```python
from build123d import *

# Parameters (mm, degrees)
F0_R     = 61.5
F1_DEPTH = 25


with BuildPart() as f1:
    # F0 (on Front) → F1 (new body)
    with BuildSketch(Plane.XZ):
        Circle(F0_R)
        with BuildLine():
            ThreePointArc((-28.054004, -53.546012), (-13.904054, -56.461066), (0, -52.537306))
            ThreePointArc((0, -52.537306), (13.904054, -56.461066), (28.054004, -53.546012))
            ThreePointArc((28.054004, -53.546012), (0, -60.45), (-28.054004, -53.546012))
        make_face(mode=Mode.SUBTRACT)
        with BuildLine():
            ThreePointArc((-44.487497, -26.839569), (-29.986229, -30.499997), (-15.488273, -26.826475))
            ThreePointArc((-15.488273, -26.826475), (-11.420658, -41.218834), (-1, -51.947086))
            ThreePointArc((-1, -51.947086), (-29.75, -51.528512), (-44.487497, -26.839569))
        make_face(mode=Mode.SUBTRACT)
        with BuildLine():
            ThreePointArc((0, -51.382534), (-10.404205, -40.976641), (-14.487497, -26.839569))
            ThreePointArc((-14.487497, -26.839569), (0, -30.5), (14.487497, -26.839569))
            ThreePointArc((14.487497, -26.839569), (10.404205, -40.976641), (0, -51.382534))
        make_face(mode=Mode.SUBTRACT)
        with BuildLine():
            ThreePointArc((-60.399208, -2.477526), (-55.848744, -16.189269), (-45.498641, -26.268653))
            ThreePointArc((-45.498641, -26.268653), (-41.94469, -40.271797), (-32.345204, -51.068486))
            ThreePointArc((-32.345204, -51.068486), (-52.351236, -30.225), (-60.399208, -2.477526))
        make_face(mode=Mode.SUBTRACT)
        with BuildLine():
            ThreePointArc((-45.487042, 25.091798), (-41.402951, 10.71203), (-30.976545, 0))
            ThreePointArc((-30.976545, 0), (-41.406887, -10.718838), (-45.487497, -25.107518))
            ThreePointArc((-45.487497, -25.107518), (-59.487041, -0.007733), (-45.487042, 25.091798))
        make_face(mode=Mode.SUBTRACT)
        with BuildLine():
            ThreePointArc((-44.498586, -25.691944), (-40.689081, -11.47831), (-30.487497, -0.873244))
            ThreePointArc((-30.487497, -0.873244), (-26.409976, -15.256598), (-15.987047, -25.974321))
            ThreePointArc((-15.987047, -25.974321), (-30.279198, -29.50655), (-44.498586, -25.691944))
        make_face(mode=Mode.SUBTRACT)
        with BuildLine():
            ThreePointArc((-29.487497, -0.858807), (-17.326184, -4.430401), (-4.76314, -2.75))
            ThreePointArc((-4.76314, -2.75), (-12.499932, -12.789714), (-15.487497, -25.107518))
            ThreePointArc((-15.487497, -25.107518), (-25.547749, -14.75), (-29.487497, -0.858807))
        make_face(mode=Mode.SUBTRACT)
        with BuildLine():
            ThreePointArc((-14.473642, -25.099514), (-10.534797, -11.238761), (-0.500455, -0.897245))
            ThreePointArc((-0.500455, -0.897245), (-4.439299, -14.757998), (-14.473642, -25.099514))
        make_face(mode=Mode.SUBTRACT)
        with BuildLine():
            ThreePointArc((1, -51.947086), (11.420658, -41.218834), (15.488273, -26.826475))
            ThreePointArc((15.488273, -26.826475), (29.986229, -30.499997), (44.487497, -26.839569))
            ThreePointArc((44.487497, -26.839569), (29.75, -51.528512), (1, -51.947086))
        make_face(mode=Mode.SUBTRACT)
        with BuildLine():
            ThreePointArc((-14, -25.966324), (-4.826252, -17.220116), (0, -5.5))
            ThreePointArc((0, -5.5), (4.826252, -17.220116), (14, -25.966324))
            ThreePointArc((14, -25.966324), (0, -29.5), (-14, -25.966324))
        make_face(mode=Mode.SUBTRACT)
        with BuildLine():
            ThreePointArc((14.486594, -25.091517), (4.452251, -14.75), (0.513406, -0.889245))
            ThreePointArc((0.513406, -0.889245), (10.547749, -11.230762), (14.486594, -25.091517))
        make_face(mode=Mode.SUBTRACT)
        with BuildLine():
            ThreePointArc((28.973189, 0), (15, -3.519238), (1.026811, 0))
            ThreePointArc((1.026811, 0), (15, 3.519238), (28.973189, 0))
        make_face(mode=Mode.SUBTRACT)
        with BuildLine():
            ThreePointArc((15.487497, -25.107518), (12.499932, -12.789714), (4.76314, -2.75))
            ThreePointArc((4.76314, -2.75), (17.326184, -4.430401), (29.487497, -0.858807))
            ThreePointArc((29.487497, -0.858807), (25.547749, -14.75), (15.487497, -25.107518))
        make_face(mode=Mode.SUBTRACT)
        with BuildLine():
            ThreePointArc((44.498579, -25.691267), (30.28471, -29.498626), (16, -25.966324))
            ThreePointArc((16, -25.966324), (26.413775, -15.25), (30.487497, -0.873244))
            ThreePointArc((30.487497, -0.873244), (40.688914, -11.478015), (44.498579, -25.691267))
        make_face(mode=Mode.SUBTRACT)
        with BuildLine():
            ThreePointArc((32.345204, -51.068486), (41.94469, -40.271797), (45.498641, -26.268653))
            ThreePointArc((45.498641, -26.268653), (55.848744, -16.189269), (60.399208, -2.477526))
            ThreePointArc((60.399208, -2.477526), (52.351236, -30.225), (32.345204, -51.068486))
        make_face(mode=Mode.SUBTRACT)
        with BuildLine():
            ThreePointArc((-32.345204, 51.068486), (-41.94469, 40.271797), (-45.498641, 26.268653))
            ThreePointArc((-45.498641, 26.268653), (-55.848744, 16.189269), (-60.399208, 2.477526))
            ThreePointArc((-60.399208, 2.477526), (-52.351236, 30.225), (-32.345204, 51.068486))
        make_face(mode=Mode.SUBTRACT)
        with BuildLine():
            ThreePointArc((-44.498426, 25.676034), (-30.286966, 29.490471), (-16.000887, 25.965778))
            ThreePointArc((-16.000887, 25.965778), (-26.414035, 15.249549), (-30.487497, 0.873244))
            ThreePointArc((-30.487497, 0.873244), (-40.685169, 11.471382), (-44.498426, 25.676034))
        make_face(mode=Mode.SUBTRACT)
        with BuildLine():
            ThreePointArc((-15.487497, 25.107518), (-12.499932, 12.789714), (-4.76314, 2.75))
            ThreePointArc((-4.76314, 2.75), (-17.326184, 4.430401), (-29.487497, 0.858807))
            ThreePointArc((-29.487497, 0.858807), (-25.547749, 14.75), (-15.487497, 25.107518))
        make_face(mode=Mode.SUBTRACT)
        with BuildLine():
            ThreePointArc((-28.973189, 0), (-15, 3.519238), (-1.026811, 0))
            ThreePointArc((-1.026811, 0), (-15, -3.519238), (-28.973189, 0))
        make_face(mode=Mode.SUBTRACT)
        with BuildLine():
            ThreePointArc((-14.486594, 25.091517), (-4.443107, 14.74859), (-0.500455, 0.881244))
            ThreePointArc((-0.500455, 0.881244), (-10.543942, 11.224172), (-14.486594, 25.091517))
        make_face(mode=Mode.SUBTRACT)
        with BuildLine():
            ThreePointArc((-1, 51.947086), (-11.420658, 41.218834), (-15.488273, 26.826475))
            ThreePointArc((-15.488273, 26.826475), (-29.986229, 30.499997), (-44.487497, 26.839569))
            ThreePointArc((-44.487497, 26.839569), (-29.75, 51.528512), (-1, 51.947086))
        make_face(mode=Mode.SUBTRACT)
        with BuildLine():
            ThreePointArc((-2e-06, 51.382535), (10.404204, 40.976642), (14.487497, 26.839569))
            ThreePointArc((14.487497, 26.839569), (0, 30.5), (-14.487497, 26.839569))
            ThreePointArc((-14.487497, 26.839569), (-10.404206, 40.976641), (-2e-06, 51.382535))
        make_face(mode=Mode.SUBTRACT)
        with BuildLine():
            ThreePointArc((14.486594, 25.091517), (10.547749, 11.230762), (0.513406, 0.889245))
            ThreePointArc((0.513406, 0.889245), (4.452251, 14.75), (14.486594, 25.091517))
        make_face(mode=Mode.SUBTRACT)
        with BuildLine():
            ThreePointArc((29.487497, 0.858807), (17.326184, 4.430401), (4.76314, 2.75))
            ThreePointArc((4.76314, 2.75), (12.499932, 12.789714), (15.487497, 25.107518))
            ThreePointArc((15.487497, 25.107518), (25.547749, 14.75), (29.487497, 0.858807))
        make_face(mode=Mode.SUBTRACT)
        with BuildLine():
            ThreePointArc((44.498579, 25.691267), (40.688914, 11.478016), (30.487496, 0.873246))
            ThreePointArc((30.487496, 0.873246), (26.413774, 15.250001), (16, 25.966324))
            ThreePointArc((16, 25.966324), (30.28471, 29.498626), (44.498579, 25.691267))
        make_face(mode=Mode.SUBTRACT)
        with BuildLine():
            ThreePointArc((-14, 25.966324), (0, 29.5), (14, 25.966324))
            ThreePointArc((14, 25.966324), (4.826252, 17.220116), (0, 5.5))
            ThreePointArc((0, 5.5), (-4.826252, 17.220116), (-14, 25.966324))
        make_face(mode=Mode.SUBTRACT)
        with BuildLine():
            ThreePointArc((45.487497, -25.107518), (41.406887, -10.718838), (30.976545, 0))
            ThreePointArc((30.976545, 0), (41.406887, 10.718838), (45.487497, 25.107518))
            ThreePointArc((45.487497, 25.107518), (59.5, 0), (45.487497, -25.107518))
        make_face(mode=Mode.SUBTRACT)
        with BuildLine():
            ThreePointArc((60.399208, 2.477526), (55.848744, 16.189269), (45.498641, 26.268653))
            ThreePointArc((45.498641, 26.268653), (41.94469, 40.271797), (32.345204, 51.068486))
            ThreePointArc((32.345204, 51.068486), (52.351236, 30.225), (60.399208, 2.477526))
        make_face(mode=Mode.SUBTRACT)
        with BuildLine():
            ThreePointArc((44.487497, 26.839569), (29.986229, 30.499997), (15.488273, 26.826475))
            ThreePointArc((15.488273, 26.826475), (11.420657, 41.218835), (0.999998, 51.947088))
            ThreePointArc((0.999998, 51.947088), (29.75, 51.528514), (44.487497, 26.839569))
        make_face(mode=Mode.SUBTRACT)
        with BuildLine():
            ThreePointArc((28.054004, 53.546012), (13.904054, 56.461066), (0, 52.537306))
            ThreePointArc((0, 52.537306), (-13.904054, 56.461066), (-28.054004, 53.546012))
            ThreePointArc((-28.054004, 53.546012), (0, 60.45), (28.054004, 53.546012))
        make_face(mode=Mode.SUBTRACT)
    extrude(amount=F1_DEPTH)


solid = f1.part
```
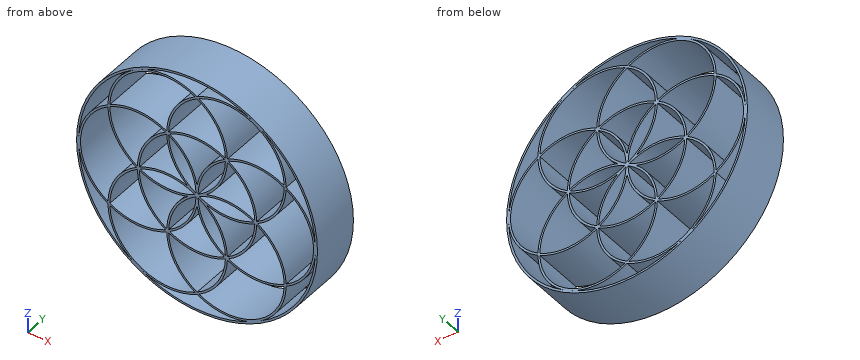
The listing builds one solid part. Answer for the finished solid, in the listing's coordinates (mm). Coordinates: 2 decimals unless noted, no trailing zeros. Loops run counter-clockwise (first coordinate to the right, second up) from the corner with the lowest first, then second, coordinate; pieces in that order, holes last. Notation, with made-up numbers: M 11.25,21.5 L 57.25,21.5 A13 ccw 57.25,46.5 Z; hole C 8,88 d7. An arc over 180 degrees is marked long. Answer as a JSON object with one key per item and string values. Group by question number.
Item 1: Section D-D (z = -41) is taken. Write down the section's boundary in (x, y).
Item 2: Section C-C (x = 53.5) is taken. Write down the section's boundary in (y, z), and give its area (3 significant figures).
Item 3: Section B-B (x = 37) is taken. Give the number of separate pieces and of enclosed holes in the cut face, and give its area (3 significant figures).
Item 4: Section A-A (z = 46) is taken. Write down the section's boundary in (x, y).
Item 5: Consider L1, parallel to X at y = -10.5, z = 47; L2, parallel to Z at x = -50, y = -10.5; L3, parallel to Z at x = -48, y = -23. Determine where each line is inside the solid, lowest interval first.
Item 6: Each of these flat-tipped pins is pushed along its axis until it touches: P1, Ø12, axis at y = -11.5, z = -14.5, coming from the -X side; P2, Ø10, axis at y = -18, z = -46, coming from the -X side; P3, Ø6, axis at y = -3.5, z = 33, coming from the -X side. Where does it stop, or does it pass through?
Solved:
{
 "1": {"outline": "M -45.84,-25 L -44.42,-25 L -44.42,0 L -45.84,0 Z; M -41.55,-25 L -40.39,-25 L -40.39,0 L -41.55,0 Z; M -11.55,-25 L -10.39,-25 L -10.39,0 L -11.55,0 Z; M 10.39,-25 L 11.55,-25 L 11.55,0 L 10.39,0 Z; M 40.39,-25 L 41.55,-25 L 41.55,0 L 40.39,0 Z; M 44.42,-25 L 45.84,-25 L 45.84,0 L 44.42,0 Z"},
 "2": {"outline": "M -25,-30.33 L 0,-30.33 L 0,-28.14 L -25,-28.14 Z; M -25,-19.44 L 0,-19.44 L 0,-17.83 L -25,-17.83 Z; M -25,17.83 L 0,17.83 L 0,19.44 L -25,19.44 Z; M -25,28.14 L 0,28.14 L 0,30.33 L -25,30.33 Z", "area": "190 mm2"},
 "3": {"separate pieces": "8", "enclosed holes": "0", "area": "265 mm2"},
 "4": {"outline": "M -40.82,-25 L -39.22,-25 L -39.22,0 L -40.82,0 Z; M -38.01,-25 L -36.67,-25 L -36.67,0 L -38.01,0 Z; M -8.01,-25 L -6.67,-25 L -6.67,0 L -8.01,0 Z; M 6.67,-25 L 8.01,-25 L 8.01,0 L 6.67,0 Z; M 36.67,-25 L 38.01,-25 L 38.01,0 L 36.67,0 Z; M 39.22,-25 L 40.82,-25 L 40.82,0 L 39.22,0 Z"},
 "5": {"L1": "x = -39.66 to -38.02, -37.1 to -35.7, -7.1 to -5.7, 5.7 to 7.1, 35.7 to 37.1, 38.02 to 39.66", "L2": "z = -35.81 to -33.97, -23.03 to -21.68, 21.67 to 23.03, 33.97 to 35.81", "L3": "z = -38.45 to -36.75, -24.62 to -23.37, 23.35 to 24.62, 36.75 to 38.45"},
 "6": {"P1": "stops at x = -60.91", "P2": "stops at x = -45.84", "P3": "stops at x = -53.69"}
}
